```python
from build123d import *

# Parameters (mm, degrees)
SKETCH1_R           = 5
BOSS_EXTRUDE1_DEPTH = 15
FILLET1_R           = 290
SKETCH3_R           = 2.5
CUT_EXTRUDE2_DEPTH  = 5


with BuildPart() as part:
    # Sketch1 → Boss-Extrude1 (new body)
    with BuildSketch(Plane(origin=(0, 0, 0), x_dir=(0, 0, -1), z_dir=(1, 0, 0))):
        with BuildLine():
            Line((-4.221556886, 7.5), (22.866991249, 12.5))
            Line((22.866991249, 12.5), (22.866991249, -12.5))
            Line((22.866991249, -12.5), (-4.221556886, -7.5))
            ThreePointArc((-4.221556886, -7.5), (-11.721556886, 0), (-4.221556886, 7.5))
        make_face()
        with Locations((-4.221556886, 0)):
            Circle(SKETCH1_R, mode=Mode.SUBTRACT)
    extrude(amount=BOSS_EXTRUDE1_DEPTH)

    # Fillet1
    fillet1_edges = [part.edges().sort_by_distance(p)[0] for p in [
        (7.5, -7.5, 4.221556886),
        (7.5, 7.5, 4.221556886),
    ]]
    fillet(fillet1_edges, radius=FILLET1_R)

    # Sketch3 → Cut-Extrude2 (cut)
    with BuildSketch(Plane(origin=(0, 0, -22.866991249), x_dir=(-1, 0, 0), z_dir=(0, 0, -1))):
        with Locations((-7.5, 0)):
            Circle(SKETCH3_R)
    extrude(amount=-CUT_EXTRUDE2_DEPTH, mode=Mode.SUBTRACT)


solid = part.part
```
The model under review builds one solid part; all positions refer to its coordinate system, in mm. A direction names the side the tool comes from. Round coordinates to 2 decimals unless told otherwise and drop trailing zeros. Loops run counter-clockwise (first coordinate to the right, second up) from the corner with the lowest first, then second, coordinate; pieces in that order, holes last.
Item 1: Take a section at D-D (y = -3.5). Write out the cut boundary in (x, z).
Determined:
outline: (0, -22.87) - (15, -22.87) - (15, 0.65) - (0, 0.65) - close; (0, 7.79) - (15, 7.79) - (15, 10.85) - (0, 10.85) - close
Item 2: For faces 5 (the face through (7.605, 8.094, 1.169)), 6 (the face through (8, 0, -17.867)), list the 3-axis set-ups (+Z, -Z, +X, -X, +Y, -Y) from which the entire face can be reached by the end or side of a thin tool; tool diameter is ignored.
Determined:
face 5: +Z, +X, -X, +Y
face 6: -Z
Item 3: Clearance check with flat-ended pins moving along their axes: pin 1 Ø8 at (y, z) = (0, 4.22) entering from -X; pin 2 Ø10 at (y, z) = (-6.5, 4.5) entering from -X; pin 3 Ø2.5 at (x, y) = (7.5, 1) entering from -Z; pin 4 Ø3 at (x, z) = (13, 4) entering from -Y. State where each tip first meets the part, or that it passes through.
Determined:
pin 1: passes through
pin 2: stops at x = 0
pin 3: stops at z = -17.87
pin 4: stops at y = -7.87
Item 4: Take a section at B-B (y = 0). Write out the cut boundary in (x, z).
Determined:
outline: (0, -22.87) - (5, -22.87) - (5, -17.87) - (10, -17.87) - (10, -22.87) - (15, -22.87) - (15, -0.78) - (0, -0.78) - close; (0, 9.22) - (15, 9.22) - (15, 11.72) - (0, 11.72) - close
Item 5: Take a section at C-C (x = 7.5). Write out the cut boundary in (y, z).
Determined:
outline: (-12.5, -22.87) - (-2.5, -22.87) - (-2.5, -17.87) - (2.5, -17.87) - (2.5, -22.87) - (12.5, -22.87) - (8.82, -2.91) arc R290 cw to (7.41, 5.37) arc R7.5 ccw to (-7.41, 5.37) arc R290 cw to (-8.82, -2.91) - close; hole circle Ø10 at (0, 4.22)
Item 6: Take a section at A-A (x = 11.75). Write out the cut boundary in (y, z), then the cut area to 3 significant figures.
Determined:
outline: (-12.5, -22.87) - (12.5, -22.87) - (8.82, -2.91) arc R290 cw to (7.41, 5.37) arc R7.5 ccw to (-7.41, 5.37) arc R290 cw to (-8.82, -2.91) - close; hole circle Ø10 at (0, 4.22)
area: 552 mm2
Item 7: For line 1 (Z direction, x = 5.75, y = -4.25); line 2 (X direction, y = -2, z = -19); line 3 (Y direction, x = 5, z = 7), list the stretches that pass through material, from the lowest coordinate up.
Determined:
line 1: z = -22.87 to 1.59, 6.86 to 10.4
line 2: x = 0 to 6, 9 to 15
line 3: y = -6.97 to -4.16, 4.16 to 6.97
Item 8: Mouldability with a two-part tool opening along Y and no side actions: class faces 1 (the face through (7.605, -8.074, 1.284)), 2 (the face through (10, 0, -20)), 3 (the face through (7.4, 1.5, -0.55)), 4 (the face through (7, 3, -22.867)) as released by +Y, released by -Y, zero draft, split by the parting line, or undercut.
Determined:
face 1: released by -Y
face 2: undercut
face 3: undercut
face 4: zero draft
